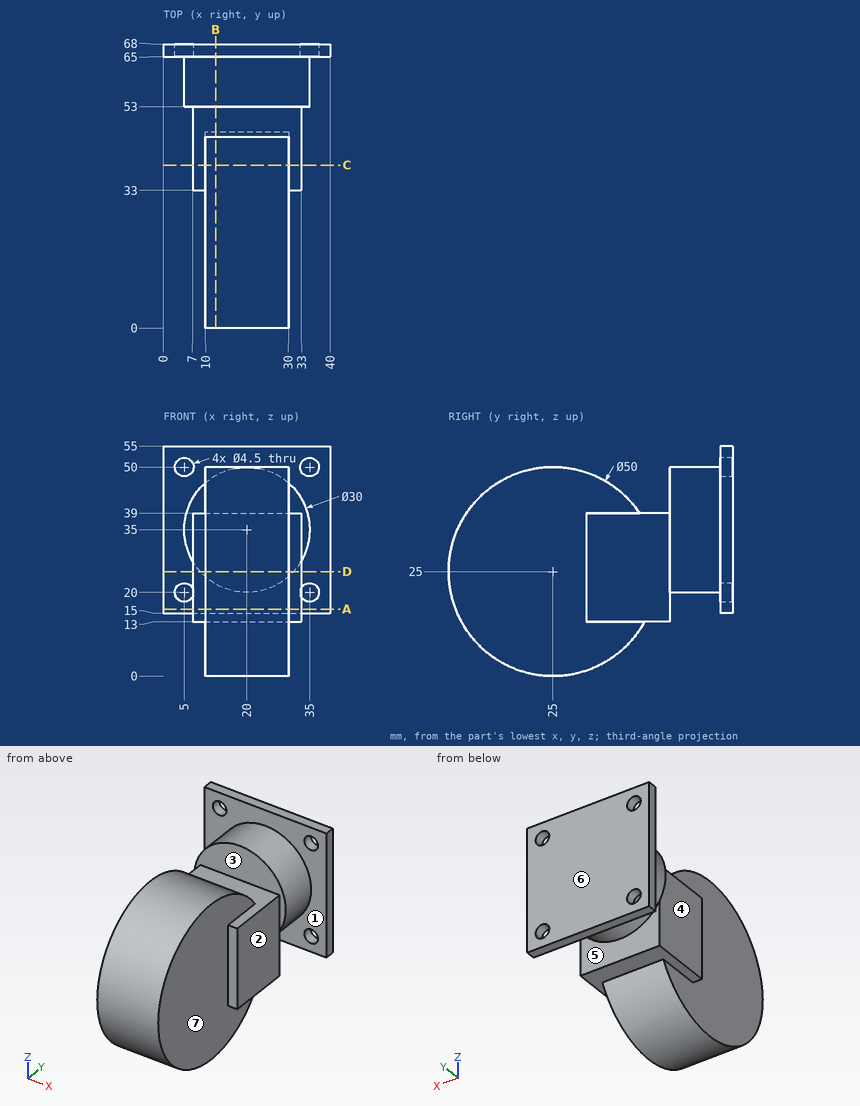
Design review of the part shown in the three views and the two pictorial views. Dimensions are in mm from the part's minimum x, y and z. A direction names the side the tool comes from. Coordinates: 2 decimals unless noted, no trailing zeros. Loops run counter-clockwise (first coordinate to the right, second up) from the corner with the lowest first, then second, coordinate; pieces in that order, holes last. Notation, with made-up numbers: (6.5, -28.5) - (55.5, -28.5) arc R21 cw to (55.5, -13.5) - close; hole circle Ø6 at (63.25, -12). An arc over 180 degrees is marked (long way). Use a Markdown table: item, result. Add a question column.
Item 1: Insertion check: pin 1 Ø3.5 at (x, z) = (35, 50) entering from -Y; pin 2 Ø1 at (y, z) = (43.5, 17) entering from -X; pin 3 Ø1.5 at (x, z) = (5.5, 31.5) entering from -Y; pin 4 Ø1 at (x, y) = (28.5, 40) entering from +Z. Each pin has a flat end and moves straight along its axis. Give the tip position at first contact, or say it passes through.
Item 2: We need section D-D (z = 25). Give the boundary of the cut face in (x, y), and give its area (3 significant figures).
Item 3: We need section B-B (x = 12.5). Give the boundary of the cut face in (y, z).
Item 4: Mouldability with a two-part tool opening along Y and no side actions: class the marked faces 5, 6 and 7 as pulls with the +Y half, pulls with the -Y half, needs draft (parallel to the pull), parting line crosses it, or undercut.
Item 5: For line 1 (X direction, y = 66.95, z = 50); line 2 (X direction, y = 31.5, z = 44); line 3 (Z direction, x = 20, y = 5), list the stretches that pass through material, from the lowest coordinate up.
Item 6: We need section A-A (z = 16). Give the boundary of the cut face in (x, y), and give its area (3 significant figures).
Item 7: Tool access review of the marked faces 1, 2, 3 and 4: name each direction out of +Z, -Z, +X, -X, +Y, -Y from which nothing blocks a thin tool from reaching the whole face with its end or side.
Item 8: We need section C-C (y = 39). Give the boundary of the cut face in (x, z).
Results list:
| question | item | result |
|---|---|---|
| 1 | pin 1 | passes through |
| 1 | pin 2 | stops at x = 7 |
| 1 | pin 3 | stops at y = 53 |
| 1 | pin 4 | stops at z = 45.37 |
| 2 | outline | (0, 65) - (8.82, 65) - (8.82, 53) - (7, 53) - (7, 33) - (10, 33) - (10, 0) - (30, 0) - (30, 33) - (33, 33) - (33, 53) - (31.18, 53) - (31.18, 65) - (40, 65) - (40, 68) - (0, 68) - close |
| 2 | area | 1,570 mm^2 |
| 3 | outline | (45.71, 39) arc R25 ccw (long way) to (46.93, 13) - (53, 13) - (53, 22.01) - (65, 22.01) - (65, 15) - (68, 15) - (68, 55) - (65, 55) - (65, 47.99) - (53, 47.99) - (53, 39) - close |
| 4 | face 5 | undercut |
| 4 | face 6 | pulls with the +Y half |
| 4 | face 7 | needs draft |
| 5 | line 1 | x = 0 to 2.75, 7.25 to 32.75, 37.25 to 40 |
| 5 | line 2 | x = 10 to 30 |
| 5 | line 3 | z = 10 to 40 |
| 6 | outline | (0, 65) - (40, 65) - (40, 68) - (0, 68) - close; (7, 33) - (10, 33) - (10, 1.68) - (30, 1.68) - (30, 33) - (33, 33) - (33, 53) - (7, 53) - close |
| 6 | area | 1,270 mm^2 |
| 7 | face 1 | none |
| 7 | face 2 | +Z, -Z, +X, -Y |
| 7 | face 3 | +Z |
| 7 | face 4 | +Z, -Z, -X, -Y |
| 8 | outline | (7, 13) - (10, 13) - (10, 4.29) - (30, 4.29) - (30, 13) - (33, 13) - (33, 39) - (30, 39) - (30, 45.71) - (10, 45.71) - (10, 39) - (7, 39) - close |
